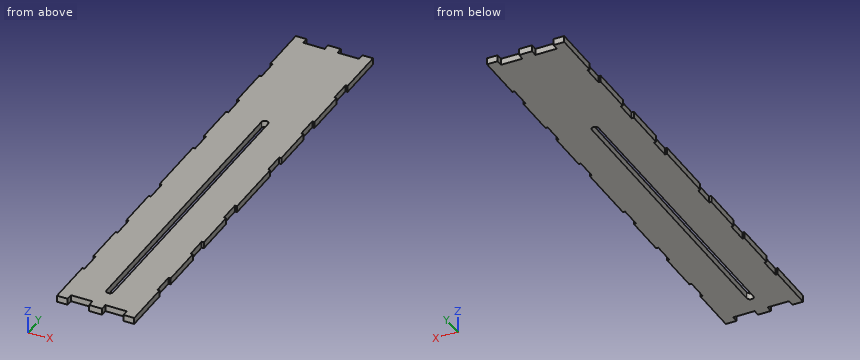
from build123d import *

# Parameters (mm, degrees)
SKETCH1_W           = 34
SKETCH1_H           = 210
SKETCH1_W_2         = 1
SKETCH1_H_2         = 20
SKETCH1_H_3         = 30
SKETCH1_W_3         = 6
SKETCH1_H_4         = 3
BOSS_EXTRUDE1_DEPTH = 3
CUT_EXTRUDE1_DEPTH  = 216.877279953


with BuildPart() as part:
    # Sketch1 → Boss-Extrude1 (new body)
    with BuildSketch(Plane.XY):
        with Locations((17, 105)):
            Rectangle(SKETCH1_W, SKETCH1_H)
        with Locations((34.5, 200)):
            Rectangle(SKETCH1_W_2, SKETCH1_H_2)
        with Locations((-0.5, 200)):
            Rectangle(SKETCH1_W_2, SKETCH1_H_2)
        with Locations((-0.5, 170)):
            Rectangle(SKETCH1_W_2, SKETCH1_H_2)
        with Locations((34.5, 170)):
            Rectangle(SKETCH1_W_2, SKETCH1_H_2)
        with Locations((34.5, 140)):
            Rectangle(SKETCH1_W_2, SKETCH1_H_2)
        with Locations((-0.5, 140)):
            Rectangle(SKETCH1_W_2, SKETCH1_H_2)
        with Locations((-0.5, 105)):
            Rectangle(SKETCH1_W_2, SKETCH1_H_3)
        with Locations((34.5, 105)):
            Rectangle(SKETCH1_W_2, SKETCH1_H_3)
        with Locations((34.5, 70)):
            Rectangle(SKETCH1_W_2, SKETCH1_H_2)
        with Locations((-0.5, 70)):
            Rectangle(SKETCH1_W_2, SKETCH1_H_2)
        with Locations((-0.5, 40)):
            Rectangle(SKETCH1_W_2, SKETCH1_H_2)
        with Locations((34.5, 40)):
            Rectangle(SKETCH1_W_2, SKETCH1_H_2)
        with Locations((34.5, 10)):
            Rectangle(SKETCH1_W_2, SKETCH1_H_2)
        with Locations((-0.5, 10)):
            Rectangle(SKETCH1_W_2, SKETCH1_H_2)
        Polygon((4, 0), (0, 0), (-1, 0), (-1, -3), (4, -3), align=None)
        with Locations((17, -1.5)):
            Rectangle(SKETCH1_W_3, SKETCH1_H_4)
        Polygon((34, 0), (30, 0), (30, -3), (35, -3), (35, 0), align=None)
        Polygon((-1, 210), (0, 210), (4, 210), (4, 213), (-1, 213), align=None)
        with Locations((17, 211.5)):
            Rectangle(SKETCH1_W_3, SKETCH1_H_4)
        Polygon((30, 213), (30, 210), (34, 210), (35, 210), (35, 213), align=None)
    extrude(amount=BOSS_EXTRUDE1_DEPTH)

    # Sketch2 → Cut-Extrude1 (cut, through all)
    with BuildSketch(Plane.XY.offset(3)):
        with BuildLine():
            Line((18.55, 150), (18.55, 10))
            ThreePointArc((18.55, 10), (17, 8.45), (15.45, 10))
            Line((15.45, 10), (15.45, 150))
            ThreePointArc((15.45, 150), (17, 151.55), (18.55, 150))
        make_face()
    extrude(amount=-CUT_EXTRUDE1_DEPTH, mode=Mode.SUBTRACT)


solid = part.part
Work out the finished part from the listing and answer in its coordinate system (mm). Give positions to 0.01 mm unless a question says otherwise; leave off trailing zeros. Order: outer loops, then holes, each group sorted by start corner. A loop starts at its lowest first (then second) coordinate and runs counter-clockwise, first axis right, second up. Notation, with made-up numbers: M 76.25,32.25 L 102.25,32.25 A9 cw 102.25,39.25 Z; hole C -36.75,87.5 d5. An arc over 180 degrees is marked long. Return JSON: item names as keys, results as strings.
Q1. Find section B-B, the plane x = 25. Write down the section's boundary in (y, z).
Answer below:
{"outline": "M 0,0 L 210,0 L 210,3 L 0,3 Z"}
Q2. Find section A-A, the plane y = 96.5. Write down the section's boundary in (x, z).
Answer below:
{"outline": "M -1,0 L 15.45,0 L 15.45,3 L -1,3 Z; M 18.55,0 L 35,0 L 35,3 L 18.55,3 Z"}
Q3. Each of these flat-tipped pins is pushed along its axis until it touches: pin 1 (0.9 mm diameter, centred on x = 23, z = 1, fed in from -Y); pin 2 (0.9 mm diameter, centred on y = 122.5, z = 2, fed in from -X); pin 3 (0.9 mm diameter, centred on y = 85.5, z = 1, fed in from +X). Where does it stop, or does it pass through?
Answer below:
{"pin 1": "stops at y = 0", "pin 2": "stops at x = 0", "pin 3": "stops at x = 34"}
Q4. Find the intervals of material crossed by line 1 along X through (y, z) = (101.5, 2.6); line 2 along X through (y, z) = (123, 0.5); line 3 along Y through (x, z) = (12.5, 2.75), in increasing order. Write a range as [from, to].
Answer below:
{"line 1": "x = [-1, 15.45], [18.55, 35]", "line 2": "x = [0, 15.45], [18.55, 34]", "line 3": "y = [0, 210]"}
